Read the model definition and answer for the solid it produces. Units are mm, in the model's axes. A direction names the side the tool comes from. Coordinates: 2 decimals unless noted, no trailing zeros. Write each loop counter-clockwise with the first axis right and the second up, starting at its lowest first coordinate (ties: lowest second). Pieces come first, ordered by that corner, then holes. Notation, with made-up numbers: M 39,71.5 L 63,71.5 A20 ccw 63,97.5 Z; hole C -38.75,-34 d3. An arc over 180 degrees is marked long. Write item = value, one per line.
from build123d import *

# Parameters (mm, degrees)
SKETCH_1_R          = 28.7
SKETCH_1_R_2        = 1.5
EXTRUDE_1_DEPTH     = 3
EXTRUDE_START       = -48
SKETCH_2_R          = 34.7
SKETCH_2_R_2        = 28.7
EXTRUDE_2_DEPTH     = 48
SKETCH_3_W          = 12
SKETCH_3_H          = 23
CUT_EXTRUDE_1_DEPTH = 96.09443105
FILLET_1_R          = 2
SKETCH_4_W          = 30
SKETCH_4_H          = 25
CUT_EXTRUDE_2_DEPTH = 96.094431221
FILLET_2_R          = 2


with BuildPart() as part:
    # 草图1 → 凸台-拉伸1 (new body)
    with BuildSketch(Plane.XY):
        Circle(SKETCH_1_R)
        with Locations((0, 19)):
            Circle(SKETCH_1_R_2, mode=Mode.SUBTRACT)
        with Locations((19, 0)):
            Circle(SKETCH_1_R_2, mode=Mode.SUBTRACT)
        with Locations((0, -19)):
            Circle(SKETCH_1_R_2, mode=Mode.SUBTRACT)
        with Locations((-19, 0)):
            Circle(SKETCH_1_R_2, mode=Mode.SUBTRACT)
    extrude(amount=EXTRUDE_1_DEPTH)

    # 草图2 → 凸台-拉伸2 (add)
    with BuildSketch(Plane.XY.offset(3).offset(EXTRUDE_START)):
        Circle(SKETCH_2_R)
        Circle(SKETCH_2_R_2, mode=Mode.SUBTRACT)
    extrude(amount=EXTRUDE_2_DEPTH)

    # 草图3 → 切除-拉伸1 (cut, through all)
    with BuildSketch(Plane(origin=(-24.536605307, 24.536605307, 0), x_dir=(0, 0, 1), z_dir=(-0.7071067811865488, 0.7071067811865464, 0))):
        with Locations((-6, 0)):
            Rectangle(SKETCH_3_W, SKETCH_3_H)
    extrude(amount=-CUT_EXTRUDE_1_DEPTH, mode=Mode.SUBTRACT)

    # 圆角1
    fillet_1_edges = [part.edges().sort_by_distance(p)[0] for p in [
        (29.00347462, -12.740018652, -12),
        (-12.740018652, 29.00347462, -12),
        (29.00347462, -12.740018652, 0),
        (-12.740018652, 29.00347462, 0),
        (12.740018652, -29.00347462, 0),
        (-29.00347462, 12.740018652, 0),
        (-29.00347462, 12.740018652, -12),
        (12.740018652, -29.00347462, -12),
    ]]
    fillet(fillet_1_edges, radius=FILLET_1_R)

    # 草图4 → 切除-拉伸2 (cut, through all)
    with BuildSketch(Plane(origin=(24.536605307, 24.536605307, 0), x_dir=(0.7071067811865487, -0.7071067811865465, 0), z_dir=(0.7071067811865465, 0.7071067811865487, 0))):
        with Locations((0, 22.5)):
            Rectangle(SKETCH_4_W, SKETCH_4_H)
    extrude(amount=-CUT_EXTRUDE_2_DEPTH, mode=Mode.SUBTRACT)

    # 圆角2
    fillet_2_edges = [part.edges().sort_by_distance(p)[0] for p in [
        (-9.107024959, -30.320228395, -35),
        (30.320228395, 9.107024959, -35),
        (-9.107024959, -30.320228395, -10),
        (30.320228395, 9.107024959, -10),
        (-30.320228395, -9.107024959, -10),
        (9.107024959, 30.320228395, -10),
        (-30.320228395, -9.107024959, -35),
        (9.107024959, 30.320228395, -35),
    ]]
    fillet(fillet_2_edges, radius=FILLET_2_R)


solid = part.part
Item 1: Which of the six approach directions +Z, -Z, +X, -X, +Y, -Y give full straight-line access (tool end or side, diameter ignored) to faces 4 (the face through (-9.86, -30.267, -34.399)), 5 (the face through (30.354, 9.141, -22.353)), 6 (the face through (-30.245, -9.882, -34.43)), 7 (the face through (12.708, -28.972, -6.056))?
Worked answers:
face_4 = -X
face_5 = +Y
face_6 = -Y
face_7 = +X
Item 2: Find section A-A (z = -32). Determine the outline of the cut face in (x, y), and give its area (3 significant figures).
Worked answers:
outline = M -32.73,-11.52 L -27.91,-6.69 A28.7 cw 6.69,27.91 L 11.52,32.73 A34.7 ccw Z; M -11.52,-32.73 A34.7 ccw 32.73,11.52 L 27.91,6.69 A28.7 cw -6.69,-27.91 Z
area = 820 mm²
Item 3: Consider line 1 along Y through (x, z) = (0, 0.9); line 2 along Y through (x, z) = (0, -15.5); line 3 along Z through (x, y) = (-20, -27.5). Determine where each line is inside the solid, lowest interval first. Write a range as from..to.
Worked answers:
line_1 = -34.7..-20.5, -17.5..17.5, 20.5..34.7
line_2 = -34.7..-28.7, 28.7..34.7
line_3 = -45..-35, -10..3
Item 4: For a pull along X with two mould halves and no side action, classify faces 1 (the face through (9.81, 30.17, -10.57)), 2 (the face through (-13.333, 28.79, -0.601)), 3 (the face through (-20.5, 0.07, 1.48)) as released by +X, released by -X, zero draft, split by the parting line, or undercut.
Worked answers:
face_1 = released by +X
face_2 = released by -X
face_3 = undercut
Item 5: Find section B-B (x = 0). Determine the outline of the cut face in (y, z).
Worked answers:
outline = M -34.7,-45 L -28.7,-45 L -28.7,0 L -20.5,0 L -20.5,3 L -34.7,3 Z; M -17.5,0 L 17.5,0 L 17.5,3 L -17.5,3 Z; M 20.5,0 L 28.7,0 L 28.7,-45 L 34.7,-45 L 34.7,3 L 20.5,3 Z
Item 6: Flat-ended cylindrical pins translate along their axes: pin 1 (6 mm diameter, centred on x = 12.5, z = -18, fed in from +Y); pin 2 (5 mm diameter, centred on x = 0, z = -6, fed in from -Y); pin 3 (4 mm diameter, centred on y = -23.5, z = -26.5, fed in from -X). Find the tip coordinate at first contact, or state that the pin passes through.
Worked answers:
pin_1 = 33.37
pin_2 = -34.7
pin_3 = 13.17
Item 7: Find section D-D (y = -19). Determine the outline of the cut face in (x, z).
Worked answers:
outline = M -29.04,-45 L -21.51,-45 L -21.51,-35 L -29.04,-35 Z; M -29.04,-10 L -21.51,-10 L -21.51,0 L -1.5,0 L -1.5,3 L -29.04,3 Z; M 1.5,0 L 29.04,0 L 29.04,3 L 1.5,3 Z; M 21.51,-45 L 29.04,-45 L 29.04,-12 L 21.51,-12 Z
